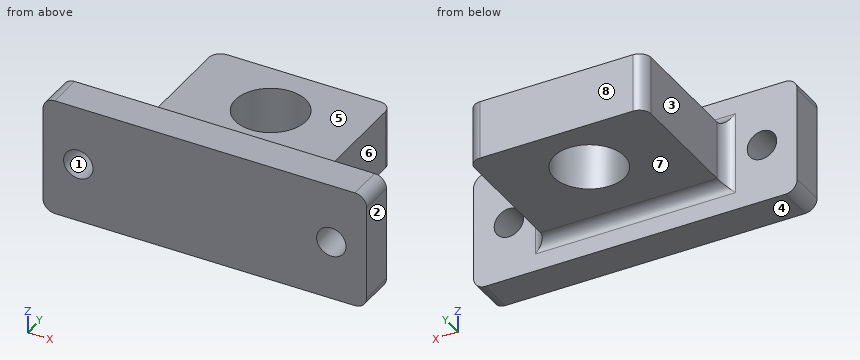
```python
from build123d import *

# Parameters (mm, degrees)
SKETCH1_W           = 30
SKETCH1_H           = 30
SKETCH1_R           = 6
BOSS_EXTRUDE1_DEPTH = 10
SKETCH2_W           = 55
SKETCH2_H           = 20
SKETCH2_R           = 2.5
BOSS_EXTRUDE2_DEPTH = 6
FILLET1_R           = 2


with BuildPart() as part:
    # Sketch1 → Boss-Extrude1 (new body)
    with BuildSketch(Plane.XY):
        with Locations((15, 15)):
            Rectangle(SKETCH1_W, SKETCH1_H)
        with Locations((15, 20)):
            Circle(SKETCH1_R, mode=Mode.SUBTRACT)
    extrude(amount=BOSS_EXTRUDE1_DEPTH)

    # Sketch2 → Boss-Extrude2 (add)
    with BuildSketch(Plane(origin=(0, 0, 0), x_dir=(-1, 0, 0), z_dir=(0, -1, 0))):
        with Locations((-15, -5)):
            Rectangle(SKETCH2_W, SKETCH2_H)
        with Locations(Location((6.5, -5, 0), (0, 0, 90))):
            Circle(SKETCH2_R, mode=Mode.SUBTRACT)
        with Locations(Location((-36.5, -5, 0), (0, 0, 270))):
            Circle(SKETCH2_R, mode=Mode.SUBTRACT)
    extrude(amount=-BOSS_EXTRUDE2_DEPTH)

    # Fillet1
    fillet1_edges = [part.edges().sort_by_distance(p)[0] for p in [
        (30, 6, 5),
        (15, 6, 10),
        (0, 6, 5),
        (42.5, 3, 15),
        (42.5, 3, -5),
        (-12.5, 3, -5),
        (-12.5, 3, 15),
        (15, 6, 0),
        (0, 30, 5),
        (30, 30, 5),
    ]]
    fillet(fillet1_edges, radius=FILLET1_R)


solid = part.part
```
Input: part model. Units: mm. Frame: model coordinates. Face numbers are marked on the shaded views. A direction names the side the tool comes from. Give positions to 0.01 mm unless a question says otherwise; leave off trailing zeros. Order: outer loops, then holes, each group sorted by start corner. A loop starts at its lowest first (then second) coordinate and runs counter-clockwise, first axis right, second up. Notation, with made-up numbers: M -39.75,25 L -27.75,25 A29 cw -27.75,63 Z; hole C 31.25,40.5 d8. An arc over 180 degrees is marked long. Return JSON: item names as keys, results as strings.
Item 1: First-contact query: P1, Ø8, axis at x = 31, z = 13, coming from the +Y side; P2, Ø1.5, axis at y = 26, z = 9, coming from the +X side; P3, Ø17.5, axis at x = 14, y = 19, coming from the -Z side. Flat tips, straight axial feed; report the tip coordinate or a pass-through.
Solutions:
{"P1": "y = 29.97", "P2": "x = 30", "P3": "z = 0"}
Item 2: Cut plane D-D (x = 6). Return loops of the section in (y, z).
Solutions:
{"outline": "M 0,-5 L 6,-5 L 6,-2 A2 cw 8,0 L 30,0 L 30,10 L 8,10 A2 cw 6,12 L 6,15 L 0,15 Z"}
Item 3: Ray query, probe 1 along X at (y, z) = (3, 5); probe 2 along Y at (x, z) = (15, 6.75); probe 3 along X at (y, z) = (19.75, 4). Return the intervals inside material, ascending.
Solutions:
{"probe 1": "-12.5 to -9, -4 to 34, 39 to 42.5", "probe 2": "0 to 14, 26 to 30", "probe 3": "0 to 9.01, 20.99 to 30"}
Item 4: Cut plane B-B (y = 20). Return loops of the section in (x, z), then the cut area to 3 significant figures.
Solutions:
{"outline": "M 0,0 L 9,0 L 9,10 L 0,10 Z; M 21,0 L 30,0 L 30,10 L 21,10 Z", "area": "180 mm^2"}
Item 5: Cut plane A-A (x = 36.5). Return loops of the section in (y, z).
Solutions:
{"outline": "M 0,-5 L 6,-5 L 6,2.5 L 0,2.5 Z; M 0,7.5 L 6,7.5 L 6,15 L 0,15 Z"}
Item 6: Cut plane C-C (z = 5). Return loops of the section in (x, y).
Solutions:
{"outline": "M -12.5,0 L -9,0 L -9,6 L -12.5,6 Z; M -4,0 L 34,0 L 34,6 L 32,6 A2 cw 30,8 L 30,28 A2 ccw 28,30 L 2,30 A2 ccw 0,28 L 0,8 A2 cw -2,6 L -4,6 Z; M 39,0 L 42.5,0 L 42.5,6 L 39,6 Z; hole C 15,20 d12"}
Item 7: Pull-direction query (X, two-part tool) for the marked faces 1, 2, 3 and 4; classes: +X half, -X half, draft (parallel to the pull), parting line (faces both ways), or undercut.
Solutions:
{"face 1": "undercut", "face 2": "+X half", "face 3": "-X half", "face 4": "draft"}
Item 8: Access query for the marked faces 5, 6, 7 and 8. Directions: +Z, -Z, +X, -X, +Y, -Y. A direction counts if a zero-diameter tool reaches every point of the face in a straight line with its end or side. Return the directions, or none.
Solutions:
{"face 5": "+Z, +X, -X, +Y", "face 6": "+Z, -Z, +X, +Y", "face 7": "-Z, +X, -X, +Y", "face 8": "+Z, -Z, +X, -X, +Y"}
